```python
from build123d import *

# Parameters (mm, degrees)
HOLE_WIZARD_M61_D        = 6.6
PATTERN_CIRCULAR_3_COUNT = 6
SKETCH_6_R               = 2.5
CUT_EXTRUDE_1_DEPTH      = 12
PATTERN_CIRCULAR_2_COUNT = 2
SKETCH_7_W               = 21.42
SKETCH_7_H               = 1.5


with BuildPart() as part:
    # Sketch 1 → Revolve 2 (revolve)
    with BuildSketch(Plane.XY, mode=Mode.PRIVATE) as revolve_2_sk:
        with BuildLine():
            Line((-12.6, 34.55), (-7.258257569, 34.55))
            ThreePointArc((-7.258257569, 34.55), (-6.8, 34.25), (-6.341742431, 34.55))
            Line((-6.341742431, 34.55), (-0.9, 34.55))
            Line((-0.9, 34.55), (-0.4, 34.05))
            Line((-0.4, 34.05), (-0.4, 24.2))
            Line((-0.4, 24.2), (-2.21470475, 24.2))
            Line((-2.21470475, 24.2), (-1.05, 21))
            Line((-1.05, 21), (-1.6, 20.799816371))
            Line((-1.6, 20.799816371), (-1.6, 17.5))
            Line((-1.6, 17.5), (-63.4, 17.5))
            Line((-63.4, 17.5), (-63.4, 19))
            Line((-63.4, 19), (-13.1, 19))
            Line((-13.1, 19), (-13.1, 34.05))
            Line((-13.1, 34.05), (-12.6, 34.55))
        make_face()
    revolve(revolve_2_sk.sketch.rotate(Axis((0, 0, 0), (-1, 0, 0)), 90), axis=Axis((0, 0, 0), (-1, 0, 0)))

    # Hole Wizard M61 (through all)
    with Locations(Plane(origin=(-0.4, 0, 0), x_dir=(0, 0, -1), z_dir=(1, 0, 0))):
        with Locations((0, 29.35)):
            hole_wizard_m61 = Hole(HOLE_WIZARD_M61_D / 2)

    # Pattern Circular 3: Hole Wizard M61 ×6 about axis
    pattern_circular_3_axis = Axis((0, 0, 0), (1, 0, 0))
    for i in range(1, PATTERN_CIRCULAR_3_COUNT):
        add(hole_wizard_m61.rotate(pattern_circular_3_axis, i * 360 / PATTERN_CIRCULAR_3_COUNT), mode=Mode.SUBTRACT)

    # Sketch 6 → Cut-Extrude 1 (cut)
    with BuildSketch(Plane(origin=(0, 0, -34.55), x_dir=(-1, 0, 0), z_dir=(0, 0, -1))):
        with Locations((-1.3, 0)):
            Circle(SKETCH_6_R)
    cut_extrude_1 = extrude(amount=-CUT_EXTRUDE_1_DEPTH, mode=Mode.SUBTRACT)

    # Pattern Circular 2: Cut-Extrude 1 ×2 about axis
    pattern_circular_2_axis = Axis((-110.150658921, 0, 0), (1, 0, 0))
    for i in range(1, PATTERN_CIRCULAR_2_COUNT):
        add(cut_extrude_1.rotate(pattern_circular_2_axis, i * 360 / PATTERN_CIRCULAR_2_COUNT), mode=Mode.SUBTRACT)

    # Sketch 7 → Cut-Revolve 1 (revolve, cut)
    with BuildSketch(Plane.XY, mode=Mode.PRIVATE) as cut_revolve_1_sk:
        with Locations((-52.69, 18.25)):
            Rectangle(SKETCH_7_W, SKETCH_7_H)
    revolve(cut_revolve_1_sk.sketch.rotate(Axis((0, 0, 0), (-1, 0, 0)), 90), axis=Axis((0, 0, 0), (-1, 0, 0)), mode=Mode.SUBTRACT)


solid = part.part
```
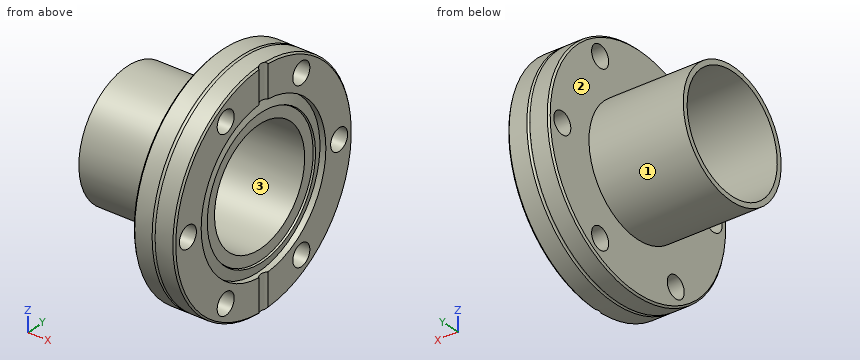
Read the model definition and answer for the solid it produces. Units are mm, in the model's axes. Face numbers are marked on the shaded views. Round coordinates to 2 decimals unless told otherwise and drop trailing zeros. Write each loop counter-clockwise with the first axis right and the second up, starting at its lowest first coordinate (ties: lowest second). Pieces come first, ordered by that corner, then holes. Notation, with made-up numbers: M 50.5,67.5 L 56.5,67.5 A20 ccw 56.5,74.5 Z; hole C -3,-36 d1. An arc over 180 degrees is marked long. One line per item, written item: value.
Q1. Find section B-B on z = 0. Count the separate pieces of the cut face and the enclosed holes in it, plus the area to 3 significant figures.
Data:
separate pieces: 4
enclosed holes: 0
area: 335 mm2
Q2. For a pull along Z with two mould halves and no side action, classify the marked faces 1, 2 and 3 as +Z half, -Z half, draft (parallel to the pull), parting line (faces both ways), or undercut.
Data:
face 1: parting line
face 2: draft
face 3: undercut
Q3. Find section A-A on x = -11. Write down the section's boundary in (y, z) (3 decimals).
Data:
outline: C 0,0 d69.1; hole C -29.35,0 d6.6; hole C -14.675,-25.418 d6.6; hole C -14.675,25.418 d6.6; hole C 0,0 d35; hole C 14.675,-25.418 d6.6; hole C 14.675,25.418 d6.6; hole C 29.35,0 d6.6
Q4. Find section D-D on x = -37.5. Write down the section's boundary in (y, z).
Data:
outline: C 0,0 d38; hole C 0,0 d35
Q5. Flat-ended cylindrical pins translate along their axes: pin 1 Ø8 at (x, y) = (-19.5, 0.5) entering from +Z; pin 2 Ø7.5 at (y, z) = (14.68, 25.42) entering from -X; pin 3 Ø7.5 at (y, z) = (14.68, -25.42) entering from +X; pin 4 Ø1 at (x, z) = (-30, 2.5) entering from -Y. Find the tip coordinate at first contact, or state that the pin passes through.
Data:
pin 1: z = 19
pin 2: x = -13.1
pin 3: x = -0.4
pin 4: y = -18.89
Q6. Straight lines are drawn through the part: line 1 (Y direction, x = -5, z = 0); line 2 (Z direction, x = -25.5, y = -0.5); line 3 (X direction, y = -5.5, z = 27.5). For each, find the intervals that lie inside material, in ascending order. Write a range as [from, to].
Data:
line 1: [-34.55, -32.65], [-26.05, -17.5], [17.5, 26.05], [32.65, 34.55]
line 2: [-18.99, -17.49], [17.49, 18.99]
line 3: [-13.1, -0.4]
